Part model, mm, in its own coordinate system. Face numbers are marked on the shaded views. A direction names the side the tool comes from. Coordinates: 2 decimals unless noted, no trailing zeros. Order: outer loops, then holes, each group sorted by start corner. A loop starts at its lowest first (then second) coordinate and runs counter-clockwise, first axis right, second up.
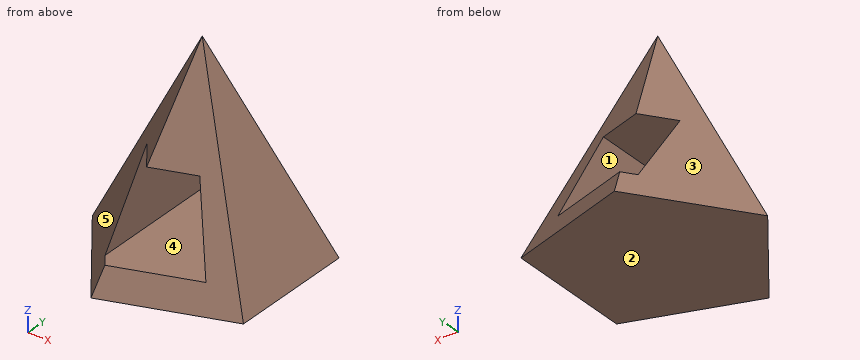
Autodesk Inventor part; units mm, degrees
ref_plane "РабПлоскость1" through (0, 0, 80) normal (0, 0, 1) x (1, 0, 0)
ref_plane "РабПлоскость2" through (0, -74.25, 0) normal (0, 1, 0) x (-1, 0, 0)
ref_plane "YZ Plane" through (0, 0, 0) normal (1, 0, 0) x (0, 1, 0)
sketch "Эскиз1" plane through (0, 0, 0) normal (0, 0, 1) x (1, 0, 0)
  line L0 (-42.5, 0) -> (-13.1332, 40.4199)
  line L1 (-13.1332, 40.4199) -> (34.3832, 24.9809)
  line L2 (34.3832, 24.9809) -> (34.3832, -24.9809)
  line L3 (34.3832, -24.9809) -> (-13.1332, -40.4199)
  line L4 (-13.1332, -40.4199) -> (-42.5, 0)
  point P0 (0, 0)
  point P1 (0, 0)
ref_plane "РабПлоскость1" through (0, 0, 80) normal (0, 0, 1) x (1, 0, 0)
sketch "Эскиз2" plane through (0, 0, 80) normal (0, 0, 1) x (1, 0, 0)
  point P0 (0, 0)
  point P1 (0, 0)
loft "Лофт1" add profiles "Эскиз1" section 2 point at (0, 0, 80)
ref_plane "РабПлоскость2" through (0, -74.25, 0) normal (0, 1, 0) x (-1, 0, 0)
sketch "Эскиз3" plane through (0, -74.25, 0) normal (0, 1, 0) x (-1, 0, 0)
  line L0 (15, 40) -> (-10, 40)
  line L1 (-10, 10) -> (15, 10)
  line L2 (15, 10) -> (15, 40)
  line L3 (-10, 40) -> (-20, 10)
  line L4 (-20, 10) -> (-10, 10)
  point P0 (0, 0)
  point P1 (0, 80)
  point P2 (42.5, 0)
  point P3 (13.1332, 0)
  point P4 (-34.3832, 0)
  dimension "d7" = 25
  dimension "d8" = 30
  dimension "d9" = 15
  dimension "d10" = 35
  dimension "d11" = 10
extrude "Выдавливание1" cut sketch "Эскиз3" along normal through all
Q1. Cut at D-D on x = 6.5. Write the cut outline in (y, z), and give its area (3 significant figures).
Results list:
outline: (-34.04, 0) - (34.04, 0) - (29.52, 10) - (-29.52, 10) - close; (-15.96, 40) - (15.96, 40) - (4.72, 64.88) - (-4.72, 64.88) - close
area: 1,150 mm2
Q2. Wall check: line 1 along Z through (x, y) = (-1, -23); line 2 along X through (y, z) = (1, 34); line 3 along Z through (x, y) = (-14, 4). Give the ranges that are in metal, low to high.
Results list:
line 1: z = 0 to 10
line 2: x = -23.71 to -15, 12 to 19.77
line 3: z = 0 to 10, 40 to 48.18
Q3. Mould opens along X. For the marked faces 1, 2 and 3 say: pulls with the +X half, pulls with the -X half, needs draft (parallel to the pull), parting line crosses it, or undercut.
Results list:
face 1: undercut
face 2: needs draft
face 3: pulls with the -X half
Q4. Cut at C-C on y = 5. Write the cut outline in (x, z).
Results list:
outline: (-38.87, 0) - (34.38, 0) - (6.88, 63.99) - (-1.62, 70.1) - close; hole (-15, 10) - (20, 10) - (10, 40) - (-15, 40) - close
Q5. Which spindle directions (+Z, -Z, +X, -X, +Y, -Y) get a long thin tool onto all of the face, cutting with end or side? Do the marked faces 4 and 5. Say none if no direction does.
Results list:
face 4: +Y, -Y
face 5: +Z, -X, -Y
Q6. Pin check, flat tips, straight feed: pin 1 Ø10 at (x, z) = (6.5, 50) entering from -Y; pin 2 Ø10 at (x, z) = (14, 13) entering from +Y. Stop position of each tip, or through.
Results list:
pin 1: stops at y = -14.23
pin 2: stops at y = 28.51
Q7. Cut at B-B on z = 37. Write the cut outline in (x, y).
Results list:
outline: (-22.84, 0) - (-15, -10.8) - (-15, 10.8) - close; (11, -15.86) - (18.48, -13.43) - (18.48, 13.43) - (11, 15.86) - close
Q8. Cut at A-A on x = -8.5. Write the cut outline in (y, z).
Results list:
outline: (-38.91, 0) - (38.91, 0) - (34.4, 10) - (-34.4, 10) - close; (-17.55, 40) - (17.55, 40) - (0, 64) - close
